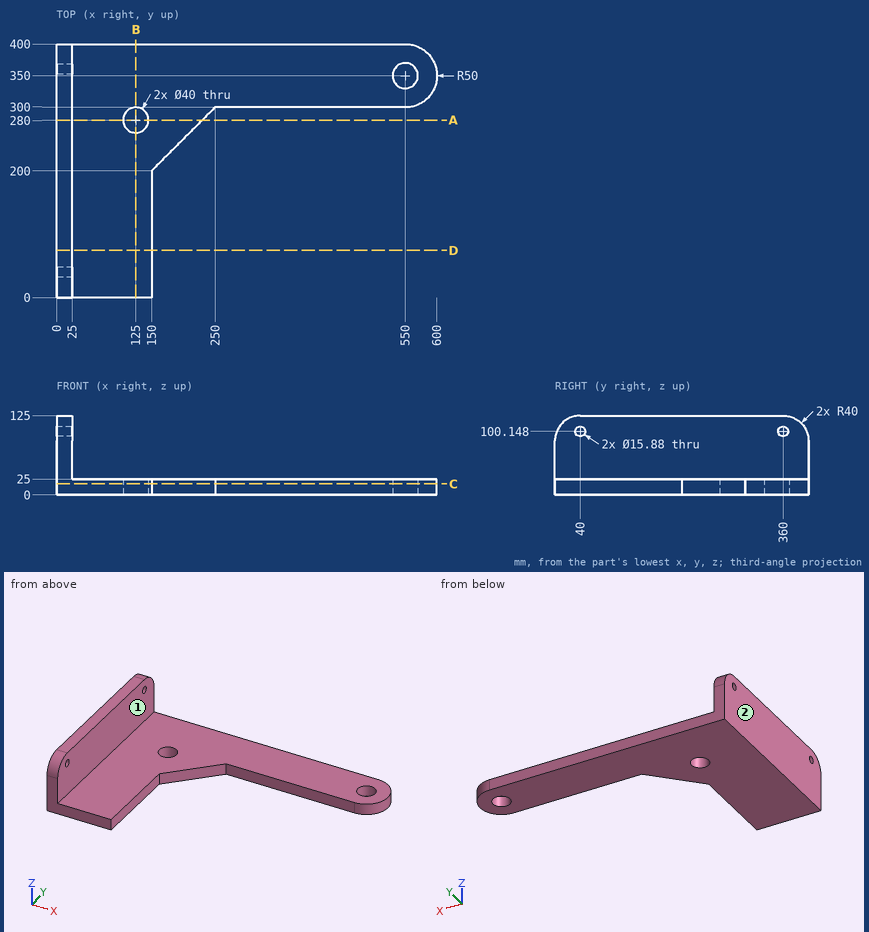
Input: dimensioned drawing with shaded views. Units: mm. Origin: part minimum x, y, z. A direction names the side the tool comes from. Give positions to 0.01 mm unless a question says otherwise; leave off trailing zeros. Write each loop counter-clockwise with the first axis right and the second up, starting at its lowest first coordinate (ties: lowest second). Pieces come first, ordered by that corner, then holes. Notation, with made-up numbers: (4, 21) -> (37, 21) arc R30 ccw to (37, 47) -> close; hole circle Ø10 at (46.25, 5). An arc over 180 degrees is marked (long way). Return JSON: item names as keys, results as strings. Group by question number.
1. Pin query (flat end, axial travel): pin 1 Ø9.5 at (y, z) = (360, 100.15) entering from -X; pin 2 Ø10 at (y, z) = (357.5, 48.5) entering from +X; pin 3 Ø12.5 at (x, z) = (333, 17.5) entering from -Y. Return the tip coordinate at first contact, or that it passes through.
2. Access query for the marked faces 1 and 2. Directions: +Z, -Z, +X, -X, +Y, -Y. A direction counts if a zero-diameter tool reaches every point of the face in a straight line with its end or side. Return the directions, or none.
3. Material intervals for line 1 (Y direction, x = 550, z = 13); line 2 (X direction, y = 252.5, z = 29.5), sorted ascending. Write a range as from..to.
4. Section D-D, the plane y = 74.5. Output: boundary loops of the cut face in (x, z).
5. Section B-B, the plane x = 125. Output: boundary loops of the cut face in (y, z), then the cut area to 3 significant figures.
6. Section A-A, the plane y = 280. Output: boundary loops of the cut face in (x, z).
7. Section C-C, the plane z = 17.5. Output: boundary loops of the cut face in (x, y), then the cut area to 3 significant figures.
Determined:
{
 "1": {"pin 1": "passes through", "pin 2": "stops at x = 25", "pin 3": "stops at y = 300"},
 "2": {"face 1": "+Z, +X, +Y, -Y", "face 2": "+Z, -Z, -X, +Y, -Y"},
 "3": {"line 1": "y = 300..330, 370..400", "line 2": "x = 0..25"},
 "4": {"outline": "(0, 0) -> (150, 0) -> (150, 25) -> (25, 25) -> (25, 125) -> (0, 125) -> close"},
 "5": {"outline": "(0, 0) -> (260, 0) -> (260, 25) -> (0, 25) -> close; (300, 0) -> (400, 0) -> (400, 25) -> (300, 25) -> close", "area": "9,000 mm2"},
 "6": {"outline": "(0, 0) -> (105, 0) -> (105, 25) -> (25, 25) -> (25, 125) -> (0, 125) -> close; (145, 0) -> (230, 0) -> (230, 25) -> (145, 25) -> close"},
 "7": {"outline": "(0, 0) -> (150, 0) -> (150, 200) -> (250, 300) -> (550, 300) arc R50 ccw to (550, 400) -> (0, 400) -> close; hole circle Ø40 at (125, 280); hole circle Ø40 at (550, 350)", "area": "106,000 mm2"}
}
